CAD build for the part. Positions are in the model's coordinates, mm. A direction names the side the tool comes from. Coordinates: 2 decimals unless noted, no trailing zeros. Write each loop counter-clockwise with the first axis right and the second up, starting at its lowest first coordinate (ties: lowest second). Pieces come first, ordered by that corner, then holes. Notation, with made-up numbers: (31, 81) - (38, 81) arc R7 cw to (38, 87) - close; hole circle Ø4 at (8.25, 22.25). An arc over 180 degrees is marked (long way). Answer in a Markdown table with one row per item. Add a question column.
Q1. Band-saw the part on D-D (x = 1.5). List the corners of the cut face in (y, z).
Q2. Band-saw the part on B-B (y = 4.75). State how many separate pieces and enclosed holes the cut face has, and give its area (3 significant figures).
Q3. Band-saw the part on C-C (y = -3). List the corners of the cut face in (x, z), and give its area (3 significant figures).
Q4. Two-plate mould, pull along X, no slides. Class faces 1 (the flat face through (3, 7, -3)), 2 (the flat face through (-2.48, 3, 0)), 3 (the flat face through (7.52, 3, 0)), 4 (the flat face through (2, 4, 1.78)): +X half, -X half, draft (parallel to the pull), parting line (faces both ways), or undercut.
Q5. Band-saw the part on A-A (y = 3). List the corners of the cut face in (x, z), and give its area (3 significant figures).
Q6. 3-axis set-ups, long thin cutter, end or side, ignore diameter. For faces 5 (the flat face through (2, 3, -3.37)), 6 (the flat face through (-1.73, 4, 0)): which of +Z, -Z, +X, -X, +Y, -Y reach the whole face in a straight line?
Q7. Pin check, flat tips, straight feed: pin 1 (1.5 mm diameter, centred on y = -0.5, z = -2, fed in from +X); pin 2 (0.5 mm diameter, centred on x = 2.5, z = 0, fed in from +Y); pin 3 (1 mm diameter, centred on x = 3.5, z = -0.5, fed in from +Y); pin 4 (0.6 mm diameter, centred on x = 4.5, z = 2.5, fed in from +Y). Stop position of each tip, or through.
Q8. Drill centre lines: line 1 along Z through (x, y) = (0, 1.5); line 2 along X through (y, z) = (6.75, 2.1); line 3 along X through (y, z) = (-2.75, -0.3). Where is each one in solid material? Low to high. Write a range as from..to.
```python
from build123d import *

# Parameters (mm, degrees)
CROQUIS1_W                   = 10
CROQUIS1_H                   = 5.9
CROQUIS1_W_2                 = 0.64
CROQUIS1_H_2                 = 0.8
SALIENTE_EXTRUIR1_DEPTH      = 1
CROQUIS2_W                   = 10
CROQUIS2_H                   = 5.9
CROQUIS2_W_2                 = 8.5
CROQUIS2_H_2                 = 4.4
SALIENTE_EXTRUIR2_DEPTH      = 6
CORTAR_EXTRUIR1_DEPTH        = 9
CORTAR_EXTRUIR2_DEPTH        = 2
SALIENTE_EXTRUIR3_DEPTH      = 6.5
SALIENTE_EXTRUIR3_DEPTH_BACK = 3.4
CROQUIS5_W                   = 0.64
CROQUIS5_H                   = 0.8


with BuildPart() as part:
    # Croquis1 → Saliente-Extruir1 (new body)
    with BuildSketch(Plane(origin=(0, 0, 0), x_dir=(1, 0, 0), z_dir=(0, 1, 0))):
        with Locations((2.52, 0.42)):
            Rectangle(CROQUIS1_W, CROQUIS1_H)
        Rectangle(CROQUIS1_W_2, CROQUIS1_H_2, mode=Mode.SUBTRACT)
        with Locations((5.04, 0)):
            Rectangle(CROQUIS1_W_2, CROQUIS1_H_2, mode=Mode.SUBTRACT)
        with Locations((2.52, 0)):
            Rectangle(CROQUIS1_W_2, CROQUIS1_H_2, mode=Mode.SUBTRACT)
    extrude(amount=SALIENTE_EXTRUIR1_DEPTH)

    # Croquis2 → Saliente-Extruir2 (add)
    with BuildSketch(Plane(origin=(0, 1, 0), x_dir=(1, 0, 0), z_dir=(0, 1, 0))):
        with Locations((2.52, 0.42)):
            Rectangle(CROQUIS2_W, CROQUIS2_H)
        with Locations((2.52, 0.42)):
            Rectangle(CROQUIS2_W_2, CROQUIS2_H_2, mode=Mode.SUBTRACT)
    extrude(amount=SALIENTE_EXTRUIR2_DEPTH)

    # Croquis3 → Cortar-Extruir1 (cut)
    with BuildSketch(Plane.ZY.offset(2.48)):
        with BuildLine():
            Line((1.78, 7), (1.78, 4.35))
            ThreePointArc((1.78, 4.35), (1.604264069, 3.925735931), (1.18, 3.75))
            Line((1.18, 3.75), (0.78, 3.75))
            Line((0.78, 3.75), (0.78, 7))
            Line((0.78, 7), (1.78, 7))
        make_face()
    extrude(amount=-CORTAR_EXTRUIR1_DEPTH, mode=Mode.SUBTRACT)

    # Croquis4 → Cortar-Extruir2 (cut)
    with BuildSketch(Plane.XY.offset(2.53)):
        with BuildLine():
            Line((-0.48, 7), (-0.48, 3.85))
            ThreePointArc((-0.48, 3.85), (-0.304264069, 3.425735931), (0.12, 3.25))
            Line((0.12, 3.25), (1.02, 3.25))
            Line((1.02, 3.25), (1.02, 7))
            Line((1.02, 7), (-0.48, 7))
        make_face()
        with BuildLine():
            Line((5.52, 7), (4.02, 7))
            Line((4.02, 7), (4.02, 3.25))
            Line((4.02, 3.25), (4.92, 3.25))
            ThreePointArc((4.92, 3.25), (5.344264069, 3.425735931), (5.52, 3.85))
            Line((5.52, 3.85), (5.52, 7))
        make_face()
    extrude(amount=-CORTAR_EXTRUIR2_DEPTH, mode=Mode.SUBTRACT)

    # Croquis5 → Saliente-Extruir3 (add, two sides: drawn at the far end of the back side and taken through both)
    with BuildSketch(Plane(origin=(0, 0, 0), x_dir=(1, 0, 0), z_dir=(0, 1, 0)).offset(-SALIENTE_EXTRUIR3_DEPTH_BACK)):
        with Locations((5.04, 0)):
            Rectangle(CROQUIS5_W, CROQUIS5_H)
        Rectangle(CROQUIS5_W, CROQUIS5_H)
        with Locations((2.52, 0)):
            Rectangle(CROQUIS5_W, CROQUIS5_H)
    extrude(amount=SALIENTE_EXTRUIR3_DEPTH + SALIENTE_EXTRUIR3_DEPTH_BACK)


solid = part.part
```
Checked values:
| question | item | result |
|---|---|---|
| 1 | outline | (0, -3.37) - (7, -3.37) - (7, -2.62) - (1, -2.62) - (1, 1.78) - (7, 1.78) - (7, 2.53) - (0, 2.53) - close |
| 2 | separate pieces | 6 |
| 2 | enclosed holes | 0 |
| 2 | area | 20.1 mm² |
| 3 | outline | (-0.32, -0.4) - (0.32, -0.4) - (0.32, 0.4) - (-0.32, 0.4) - close; (2.2, -0.4) - (2.84, -0.4) - (2.84, 0.4) - (2.2, 0.4) - close; (4.72, -0.4) - (5.36, -0.4) - (5.36, 0.4) - (4.72, 0.4) - close |
| 3 | area | 1.54 mm² |
| 4 | face 1 | draft |
| 4 | face 2 | -X half |
| 4 | face 3 | +X half |
| 4 | face 4 | undercut |
| 5 | outline | (-2.48, -3.37) - (7.52, -3.37) - (7.52, 2.53) - (-2.48, 2.53) - close; (-0.32, -0.4) - (0.32, -0.4) - (0.32, 0.4) - (-0.32, 0.4) - close; (2.2, -0.4) - (2.84, -0.4) - (2.84, 0.4) - (2.2, 0.4) - close; (4.72, -0.4) - (5.36, -0.4) - (5.36, 0.4) - (4.72, 0.4) - close; hole (-1.73, -2.62) - (6.77, -2.62) - (6.77, 1.78) - (-1.73, 1.78) - close |
| 5 | area | 23.1 mm² |
| 6 | face 5 | -Z, +X, -X, +Y, -Y |
| 6 | face 6 | +Y |
| 7 | pin 1 | stops at x = 7.52 |
| 7 | pin 2 | stops at y = 6.5 |
| 7 | pin 3 | stops at y = 1 |
| 7 | pin 4 | stops at y = 3.25 |
| 8 | line 1 | z = -3.37..-2.62, -0.4..0.4, 1.78..2.53 |
| 8 | line 2 | x = -2.48..-0.48, 1.02..4.02, 5.52..7.52 |
| 8 | line 3 | x = -0.32..0.32, 2.2..2.84, 4.72..5.36 |
